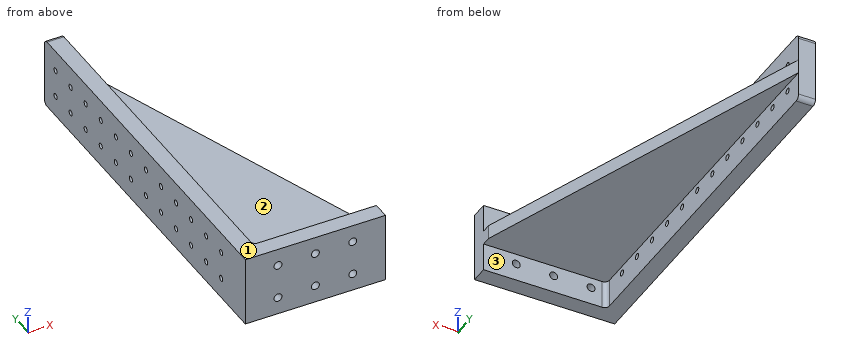
Solid Edge part; units mm, degrees
sketch "Sketch1" plane through (0, 0, 0) normal (0, 0, 1) x (1, 0, 0)
  line L0 (0, 0) -> (150, 0)
  line L1 (150, 0) -> (150, 18)
  line L2 (150, 18) -> (23, 18)
  arc A0 (23, 18) -> (18, 23) centre (23, 23) cw
  line L3 (18, 23) -> (18, 400)
  line L4 (18, 400) -> (0, 400)
  line L5 (0, 400) -> (0, 0)
extrude "ExtrudedProtrusion_1" add sketch "Sketch1" against normal blind 37.5 and the other way blind 37.5
sketch "Sketch2" plane through (0, 0, 0) normal (0, 0, 1) x (1, 0, 0)
  line L0 (0, 0) -> (150, 0)
  line L1 (150, 0) -> (150, 28)
  line L2 (150, 28) -> (18, 400)
  line L3 (18, 400) -> (0, 400)
  line L4 (0, 400) -> (0, 0)
extrude "ExtrudedProtrusion_2" add sketch "Sketch2" against normal blind 7.5 and the other way blind 7.5
sketch "Sketch3" plane through (0, 0, 0) normal (1, 0, 0) x (0, 1, 0)
  line L0 (390, 47.5) -> (390, 37.5)
  line L1 (390, 37.5) -> (395, 37.5)
  arc A0 (395, 37.5) -> (400, 32.5) centre (395, 32.5) cw
  line L2 (400, 32.5) -> (400, -32.5)
  arc A1 (400, -32.5) -> (395, -37.5) centre (395, -32.5) cw
  line L3 (395, -37.5) -> (390, -37.5)
  line L4 (390, -37.5) -> (390, -47.5)
  line L5 (390, -47.5) -> (410, -47.5)
  line L6 (410, -47.5) -> (410, 47.5)
  line L7 (410, 47.5) -> (390, 47.5)
extrude "ExtrudedCutout_1" cut sketch "Sketch3" along normal blind 18
hole "Hole_1" at (75, 0, 18.75) direction (0, 1, 0) diameter 8.5 end up to next
hole "Hole1" at (115, 0, 18.75) direction (0, 1, 0) diameter 8.5 end up to next
hole "Hole2" at (35, 0, -18.75) direction (0, 1, 0) diameter 8.5 end up to next
hole "Hole3" at (75, 0, -18.75) direction (0, 1, 0) diameter 8.5 end up to next
hole "Hole4" at (115, 0, -18.75) direction (0, 1, 0) diameter 8.5 end up to next
hole "Hole5" at (35, 0, 18.75) direction (0, 1, 0) diameter 8.5 end up to next
hole "Hole_7" at (18, 78, -15) direction (-1, 0, 0) diameter 6.1 end up to next
hole "Hole6" at (18, 108, -15) direction (-1, 0, 0) diameter 6.1 end up to next
hole "Hole7" at (18, 138, -15) direction (-1, 0, 0) diameter 6.1 end up to next
hole "Hole8" at (18, 168, -15) direction (-1, 0, 0) diameter 6.1 end up to next
hole "Hole9" at (18, 198, -15) direction (-1, 0, 0) diameter 6.1 end up to next
hole "Hole10" at (18, 228, -15) direction (-1, 0, 0) diameter 6.1 end up to next
hole "Hole11" at (18, 48, 15) direction (-1, 0, 0) diameter 6.1 end up to next
hole "Hole12" at (18, 78, 15) direction (-1, 0, 0) diameter 6.1 end up to next
hole "Hole13" at (18, 108, 15) direction (-1, 0, 0) diameter 6.1 end up to next
hole "Hole14" at (18, 138, 15) direction (-1, 0, 0) diameter 6.1 end up to next
hole "Hole15" at (18, 168, 15) direction (-1, 0, 0) diameter 6.1 end up to next
hole "Hole16" at (18, 198, 15) direction (-1, 0, 0) diameter 6.1 end up to next
hole "Hole17" at (18, 228, 15) direction (-1, 0, 0) diameter 6.1 end up to next
hole "Hole18" at (18, 258, 15) direction (-1, 0, 0) diameter 6.1 end up to next
hole "Hole19" at (18, 288, 15) direction (-1, 0, 0) diameter 6.1 end up to next
hole "Hole20" at (18, 318, 15) direction (-1, 0, 0) diameter 6.1 end up to next
hole "Hole21" at (18, 348, 15) direction (-1, 0, 0) diameter 6.1 end up to next
hole "Hole22" at (18, 378, 15) direction (-1, 0, 0) diameter 6.1 end up to next
hole "Hole23" at (18, 258, -15) direction (-1, 0, 0) diameter 6.1 end up to next
hole "Hole24" at (18, 288, -15) direction (-1, 0, 0) diameter 6.1 end up to next
hole "Hole25" at (18, 318, -15) direction (-1, 0, 0) diameter 6.1 end up to next
hole "Hole26" at (18, 348, -15) direction (-1, 0, 0) diameter 6.1 end up to next
hole "Hole27" at (18, 378, -15) direction (-1, 0, 0) diameter 6.1 end up to next
hole "Hole28" at (18, 48, -15) direction (-1, 0, 0) diameter 6.1 end up to next
Could you check a few things on this model? Use its own coordinates, in mm. Face numbers are marked on the shaded views. A direction names the side the tool comes from. Give positions to 0.01 mm unless a question says otherwise; leave off trailing zeros. Loops run counter-clockwise (first coordinate to the right, second up) from the corner with the lowest first, then second, coordinate; pieces in that order, holes last. Notation, with made-up numbers: (9.25, 3.5) - (18.25, 3.5) arc R20 ccw to (18.25, 41.5) - close; hole circle Ø11 at (6, -3). An arc over 180 degrees is marked (long way). Answer in a Markdown table with one row per item. Add a question column.
Q1. If we section it at B-B (x = 35): List the corners of the cut face in (y, z) for me.
Q2. If we section it at A-A (z = -1.5): List the corners of the cut face in (x, y) for me, plus the area to 3 significant figures.
Q3. Please list where these lines run through material, in increasing order: L1, parallel to Z at x = 13, y = 378; L2, parallel to X at y = 10.25, z = 18.75; L3, parallel to Z at x = 87.5, y = 76. Write a range as from..to.
Q4. If we section it at D-D (x = 102): List the corners of the cut face in (y, z) for me.
Q5. If we section it at C-C (x = 57): List the corners of the cut face in (y, z) for me.
Q6. Which directions (+Z, -Z, +X, -X, +Y, -Y) give clear straight access to the entire face, cutting with the end or side of a thin tool? Please do the marked faces 1, 2 and 3.
Q7. For pin 1 (5 mm diameter, centred on y = 168, z = 15, fed in from +X); pin 2 (3 mm diameter, centred on x = 120.5, z = 28, fed in from +Y); pin 3 (1.5 mm diameter, centred on y = 208.5, z = 29, fed in from +X); pin 4 (1 mm diameter, centred on x = 24, y = 181.5, fed in from +Z), each with a flat end and sliding along its axis, tell me the tip position at first contact or that it passes through.
The answers:
| question | item | result |
|---|---|---|
| 1 | outline | (0, -37.5) - (18, -37.5) - (18, -23) - (0, -23) - close; (0, -14.5) - (18, -14.5) - (18, -7.5) - (352.09, -7.5) - (352.09, 7.5) - (18, 7.5) - (18, 14.5) - (0, 14.5) - close; (0, 23) - (18, 23) - (18, 37.5) - (0, 37.5) - close |
| 2 | outline | (0, 0) - (150, 0) - (150, 28) - (18, 400) - (0, 400) - close |
| 2 | area | 35,400 mm^2 |
| 3 | L1 | z = -37.5..-18.05, -11.95..11.95, 18.05..37.5 |
| 3 | L2 | x = 0..30.75, 39.25..70.75, 79.25..110.75, 119.25..150 |
| 3 | L3 | z = -7.5..7.5 |
| 4 | outline | (0, -37.5) - (18, -37.5) - (18, -7.5) - (163.27, -7.5) - (163.27, 7.5) - (18, 7.5) - (18, 37.5) - (0, 37.5) - close |
| 5 | outline | (0, -37.5) - (18, -37.5) - (18, -7.5) - (290.09, -7.5) - (290.09, 7.5) - (18, 7.5) - (18, 37.5) - (0, 37.5) - close |
| 6 | face 1 | +Z, +X, -X, +Y, -Y |
| 6 | face 2 | +Z, +X, +Y |
| 6 | face 3 | -Z, +X, +Y |
| 7 | pin 1 | passes through |
| 7 | pin 2 | stops at y = 18 |
| 7 | pin 3 | stops at x = 18 |
| 7 | pin 4 | stops at z = 7.5 |
